Autodesk Inventor part; units mm, degrees
ref_plane "Work Plane1" through (0, 0, 2.9972) normal (0, 0, 1) x (1, 0, 0)
ref_plane "Work Plane2" through (-75, -75, -12) normal (0, 0, -1) x (0, 1, 0)
ref_plane "YZ Plane" through (0, 0, 0) normal (1, 0, 0) x (0, 1, 0)
ref_plane "Work Plane1" through (0, 0, 2.9972) normal (0, 0, 1) x (1, 0, 0)
sketch "Sketch1" plane through (0, 0, 2.9972) normal (0, 0, 1) x (1, 0, 0)
  circle A0 centre (0, 0) radius 17.4625
  circle A1 centre (0, 0) radius 32.5 construction
  circle A2 centre (0, 0) radius 45
  circle A3 centre (0, -32.5) radius 4.5
  circle A4 centre (28.1458, -16.25) radius 4.5
  circle A5 centre (28.1458, 16.25) radius 4.5
  circle A6 centre (0, 32.5) radius 4.5
  circle A7 centre (-28.1458, 16.25) radius 4.5
  circle A8 centre (-28.1458, -16.25) radius 4.5
  point P0 (0, 0)
  dimension "d1" = 65
  dimension "d0" = 34.925
  dimension "d2" = 90
  dimension "d3" = 9
  dimension "d6" = 360
extrude "Extrusion1" add sketch "Sketch1" along normal blind 8 contours A0 | A2
ref_plane "Work Plane2" through (-75, -75, -12) normal (0, 0, -1) x (0, 1, 0)
extrude "Extrusion2" add sketch "Sketch1" against normal up to surface (14.9972 mm away) contours A0
sketch "Sketch3" plane through (0, 0, 10.9972) normal (0, 0, 1) x (1, 0, 0)
  circle A0 centre (-28.1458, -16.25) radius 4.5
  circle A1 centre (-28.1458, -16.25) radius 3
  circle A2 centre (0, 32.5) radius 4.5
  circle A3 centre (0, 32.5) radius 3
  circle A4 centre (-28.1458, 16.25) radius 4.5
  circle A5 centre (-28.1458, 16.25) radius 3
  circle A6 centre (28.1458, 16.25) radius 4.5
  circle A7 centre (28.1458, 16.25) radius 3
  circle A8 centre (28.1458, -16.25) radius 4.5
  circle A9 centre (28.1458, -16.25) radius 3
  circle A10 centre (0, -32.5) radius 4.5
  circle A11 centre (0, -32.5) radius 3
  point P0 (0, 0)
  dimension "d12" = 6
  dimension "d13" = 6
  dimension "d14" = 6
  dimension "d15" = 6
  dimension "d16" = 6
  dimension "d17" = 6
extrude "Extrusion3" add sketch "Sketch3" against normal blind 2
sketch "Sketch4" plane through (0, 0, 10.9972) normal (0, 0, 1) x (1, 0, 0)
  point P0 (0, 0)
  point P1 (0, 0)
hole "Hole1" at (0, 0, 10.9972) direction (0, 0, -1) diameter 20 end through all counterbore diameter 24 counterbore depth 10
sketch "Sketch5" plane through (0, 0, 2.9972) normal (0, 0, -1) x (-1, 0, 0)
  circle A0 centre (0, 0) radius 15.7248
  circle A1 centre (0, 0) radius 18.2248
  circle A2 centre (0, 0) radius 17.4625
  point P0 (0, 0)
  dimension "d27" = 2.5
extrude "Extrusion4" add sketch "Sketch5" along normal blind 1 contours A1
properties part number "Input pin holder"
The listing builds one solid part. Answer for the finished solid, in the listing's coordinates (mm). A direction names the side the tool comes from. Coordinates: 2 decimals unless noted, no trailing zeros. Write each loop counter-clockwise with the first axis right and the second up, starting at its lowest first coordinate (ties: lowest second). Pieces come first, ordered by that corner, then holes. Notation, with made-up numbers: (-37, 44.25) - (-28, 44.25) arc R24 ccw to (-28, 71.25) - close; hole circle Ø6 at (80, -26.5). An arc over 180 degrees is marked (long way). Answer as CSV lines item,"result".
1. Find section D-D (y = 16.25). Give the vertices of the cut face in (x, z).
Computed values:
outline,"(-41.96, 3) - (-32.65, 3) - (-32.65, 9) - (-31.15, 9) - (-31.15, 11) - (-41.96, 11) - close; (-25.15, 9) - (-23.65, 9) - (-23.65, 3) - (-8.25, 3) - (-8.25, 2) - (-6.39, 2) - (-6.39, -12) - (6.39, -12) - (6.39, 2) - (8.25, 2) - (8.25, 3) - (23.65, 3) - (23.65, 9) - (25.15, 9) - (25.15, 11) - (-25.15, 11) - close; (31.15, 9) - (32.65, 9) - (32.65, 3) - (41.96, 3) - (41.96, 11) - (31.15, 11) - close"
2. Find section B-B (y = -31). Give the vertices of the cut face in (x, z).
Computed values:
outline,"(-32.62, 3) - (-4.24, 3) - (-4.24, 9) - (-2.6, 9) - (-2.6, 11) - (-32.62, 11) - close; (2.6, 9) - (4.24, 9) - (4.24, 3) - (32.62, 3) - (32.62, 11) - (2.6, 11) - close"
3. Determine the mould class of faces 1 (the cylindrical face through (-28.796, 13.321, 10.011)), 2 (the cylindrical face through (2.37, -18.07, 2.5)), 3 (the flat face through (8, -8, -12)) for opening direction X: +X half, -X half, draft (parallel to the pull), parting line (faces both ways), or undercut.
Computed values:
face 1,"undercut"
face 2,"parting line"
face 3,"draft"
4. Given P1, Ø3.5, axis at x = 0, y = 32.5, coming from the +Z side; P2, Ø8, axis at x = 0, y = -32.5, coming from the -Z side; P3, Ø10, axis at x = -26, y = -17.5, coming from the -Z side; P4, Ø6, axis at y = -18.5, z = -8, coming from the +X side, each flat-ended and moving along its own axis, determine where each tip first touches the part or whether it passes through.
Computed values:
P1,"passes through"
P2,"stops at z = 9"
P3,"stops at z = 3"
P4,"stops at x = 8.04"
5. Find section A-A (z = 7.75). Give the vertices of the cut face in (x, y), plus the area to 3 significant figures.
Computed values:
outline,"circle Ø90 at (0, 0); hole circle Ø9 at (-28.15, -16.25); hole circle Ø9 at (-28.15, 16.25); hole circle Ø24 at (0, 0); hole circle Ø9 at (0, -32.5); hole circle Ø9 at (0, 32.5); hole circle Ø9 at (28.15, -16.25); hole circle Ø9 at (28.15, 16.25)"
area,"5,530 mm²"
6. A tool of negligible diameter and unlimited length cuts with its end or side. For faces 4 (the cylindrical face through (-0.53, 11.99, 5.93)), 5 (the cylindrical face through (-28.796, -19.179, 10.011)), 6 (the flat face through (3, 34, 8.997)), from which of +Z, -Z, +X, -X, +Y, -Y can it reach the whole face along a straight path? Write none if from no direction.
Computed values:
face 4,"+Z"
face 5,"+Z, -Z"
face 6,"-Z"
7. Find section C-C (x = -7). Give the vertices of the cut face in (y, z), plus the area to 3 significant figures.
Computed values:
outline,"(-44.45, 3) - (-16.83, 3) - (-16.83, 2) - (-16, 2) - (-16, -12) - (-7.14, -12) - (-7.14, 1) - (-9.75, 1) - (-9.75, 11) - (-44.45, 11) - close; (7.14, -12) - (16, -12) - (16, 2) - (16.83, 2) - (16.83, 3) - (44.45, 3) - (44.45, 11) - (9.75, 11) - (9.75, 1) - (7.14, 1) - close"
area,"812 mm²"
8. Straight lines are drawn through the part: line 1 (Y direction, x = 0, z = 5.25); line 2 (Y direction, x = 0, z = 9.6); line 3 (Z direction, x = -16, y = 22.5). For each, find the intervals that lie inside material, in ascending order. Write a range as [from, to].
Computed values:
line 1,"y = [-45, -37], [-28, -12], [12, 28], [37, 45]"
line 2,"y = [-45, -35.5], [-29.5, -12], [12, 29.5], [35.5, 45]"
line 3,"z = [3, 11]"
